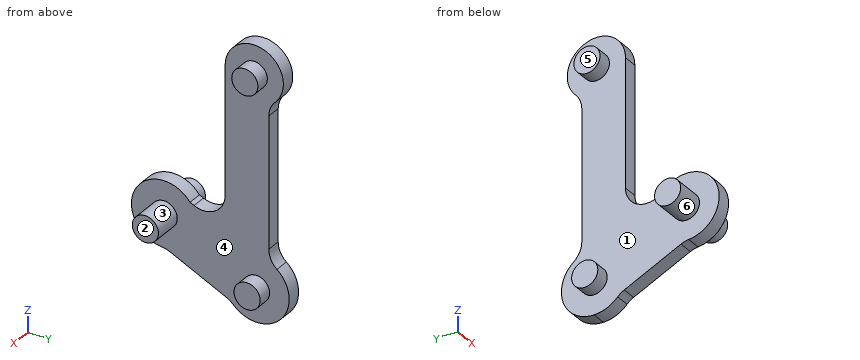
```python
from build123d import *

# Parameters (mm, degrees)
EXTRUDE_1_DEPTH     = 2
SKETCH_1_3_R        = 2
CUT_EXTRUDE_1_DEPTH = 35.66133887
FILLET_1_R          = 3
EXTRUDE_START       = -2
SKETCH_2_R          = 2
EXTRUDE_2_DEPTH     = 2
SKETCH_2_5_R        = 1.8
EXTRUDE_5_DEPTH     = 2
EXTRUDE_START_2     = -4
SKETCH_2_6_R        = 1.8
EXTRUDE_6_DEPTH     = 2
SKETCH_2_7_R        = 1.8
EXTRUDE_7_DEPTH     = 4
EXTRUDE_START_3     = -6
SKETCH_2_8_R        = 1.8
EXTRUDE_8_DEPTH     = 4


with BuildPart() as part:
    # 草图1 → 凸台-拉伸1 (new body)
    with BuildSketch(Plane(origin=(0, 0, 0), x_dir=(0, 0, -1), z_dir=(1, 0, 0))):
        with BuildLine():
            Line((-25, -6), (-25, 0))
            Line((-25, 0), (-21.535898385, 0))
            ThreePointArc((-21.535898385, 0), (-28.464101615, 0), (-25, -6))
        make_face()
        with BuildLine():
            Line((-21.535898385, 0), (-25, 0))
            Line((-25, 0), (-25, -6))
            ThreePointArc((-25, -6), (-22.171572875, -4.828427125), (-21, -2))
            ThreePointArc((-21, -2), (-21.136296695, -0.96472382), (-21.535898385, 0))
        make_face()
        with BuildLine():
            Line((-0.545176611, 0), (-21.535898385, 0))
            ThreePointArc((-21.535898385, 0), (-21.136296695, -0.96472382), (-21, -2))
            ThreePointArc((-21, -2), (-22.171572875, -4.828427125), (-25, -6))
            Line((-25, -6), (-2.797845949, -6))
            Line((-2.797845949, -6), (-0.871249866, -1.868401368))
            ThreePointArc((-0.871249866, -1.868401368), (-0.807766841, -0.916826597), (-0.545176611, 0))
        make_face()
        with BuildLine():
            ThreePointArc((8.125231148, -1.690473047), (4.486383017, 2.726360373), (-0.545176611, 0))
            Line((-0.545176611, 0), (0, 0))
            Line((0, 0), (7.250462296, -3.380946094))
            Line((7.250462296, -3.380946094), (6.37921243, -5.249347462))
            ThreePointArc((6.37921243, -5.249347462), (7.66521356, -3.67252807), (8.125231148, -1.690473047))
        make_face()
        with BuildLine():
            Line((0, 0), (-0.545176611, 0))
            ThreePointArc((-0.545176611, 0), (-0.807766841, -0.916826597), (-0.871249866, -1.868401368))
            Line((-0.871249866, -1.868401368), (0, 0))
        make_face()
        with BuildLine():
            Line((-0.871249866, -1.868401368), (-2.797845949, -6))
            Line((-2.797845949, -6), (0, -6))
            Line((0, -6), (0, -4.356499889))
            ThreePointArc((0, -4.356499889), (-0.621910323, -3.177681615), (-0.871249866, -1.868401368))
        make_face()
        with BuildLine():
            Line((0, -6), (-2.797845949, -6))
            Line((-2.797845949, -6), (-5.045405798, -10.819907651))
            ThreePointArc((-5.045405798, -10.819907651), (-0.389642338, -10.300397024), (2.205056498, -14.200853745))
            Line((2.205056498, -14.200853745), (6.37921243, -5.249347462))
            ThreePointArc((6.37921243, -5.249347462), (3.001481776, -6.147034134), (0, -4.356499889))
            Line((0, -4.356499889), (0, -6))
        make_face()
        with BuildLine():
            Line((7.250462296, -3.380946094), (0, 0))
            Line((0, 0), (0, -4.356499889))
            ThreePointArc((0, -4.356499889), (3.001481776, -6.147034134), (6.37921243, -5.249347462))
            Line((6.37921243, -5.249347462), (7.250462296, -3.380946094))
        make_face()
        with BuildLine():
            Line((0, -4.356499889), (0, 0))
            Line((0, 0), (-0.871249866, -1.868401368))
            ThreePointArc((-0.871249866, -1.868401368), (-0.621910323, -3.177681615), (0, -4.356499889))
        make_face()
        with BuildLine():
            ThreePointArc((2.205056498, -14.200853745), (-0.389642338, -10.300397024), (-5.045405798, -10.819907651))
            Line((-5.045405798, -10.819907651), (-5.916655664, -12.688309019))
            Line((-5.916655664, -12.688309019), (1.333806632, -16.069255112))
            Line((1.333806632, -16.069255112), (2.205056498, -14.200853745))
        make_face()
        with BuildLine():
            Line((-5.916655664, -12.688309019), (-5.045405798, -10.819907651))
            ThreePointArc((-5.045405798, -10.819907651), (-4.27347954, -18.418764477), (2.208575484, -14.378782065))
            ThreePointArc((2.208575484, -14.378782065), (2.207695651, -14.289800508), (2.205056498, -14.200853745))
            Line((2.205056498, -14.200853745), (1.333806632, -16.069255112))
            Line((1.333806632, -16.069255112), (-5.916655664, -12.688309019))
        make_face()
    extrude(amount=EXTRUDE_1_DEPTH)

    # 草图1<3> → 切除-拉伸1 (cut, through all)
    with BuildSketch(Plane(origin=(0, 0, 0), x_dir=(0, 0, -1), z_dir=(1, 0, 0))):
        with Locations((-25, -2)):
            Circle(SKETCH_1_3_R)
        with Locations((3.625231148, -1.690473047)):
            Circle(SKETCH_1_3_R)
        with Locations((-2.291424516, -14.378782065)):
            Circle(SKETCH_1_3_R)
    extrude(amount=CUT_EXTRUDE_1_DEPTH, mode=Mode.SUBTRACT)

    # 圆角1
    fillet_1_edges = [part.edges().sort_by_distance(p)[0] for p in [
        (1, -6, 2.797845949),
        (1, 0, 0.545176611),
        (1, -5.249347462, -6.37921243),
        (1, -14.200853745, -2.205056498),
        (1, 0, 21.535898385),
    ]]
    fillet(fillet_1_edges, radius=FILLET_1_R)

    # 草图2 → 凸台-拉伸2 (add)
    with BuildSketch(Plane(origin=(2, 0, 0), x_dir=(0, 0, -1), z_dir=(1, 0, 0)).offset(EXTRUDE_START)):
        with Locations((3.625231148, -1.690473047)):
            Circle(SKETCH_2_R)
        with Locations((-2.291424516, -14.378782065)):
            Circle(SKETCH_2_R)
        with Locations((-25, -2)):
            Circle(SKETCH_2_R)
    extrude(amount=EXTRUDE_2_DEPTH)

    # 草图2<5> → 凸台-拉伸5 (add)
    with BuildSketch(Plane(origin=(2, 0, 0), x_dir=(0, 0, -1), z_dir=(1, 0, 0))):
        with Locations((-25, -2)):
            Circle(SKETCH_2_5_R)
        with Locations((3.625231148, -1.690473047)):
            Circle(SKETCH_2_5_R)
    extrude(amount=EXTRUDE_5_DEPTH)

    # 草图2<6> → 凸台-拉伸6 (add)
    with BuildSketch(Plane(origin=(2, 0, 0), x_dir=(0, 0, -1), z_dir=(1, 0, 0)).offset(EXTRUDE_START_2)):
        with Locations((-25, -2)):
            Circle(SKETCH_2_6_R)
        with Locations((3.625231148, -1.690473047)):
            Circle(SKETCH_2_6_R)
    extrude(amount=EXTRUDE_6_DEPTH)

    # 草图2<7> → 凸台-拉伸7 (add)
    with BuildSketch(Plane(origin=(2, 0, 0), x_dir=(0, 0, -1), z_dir=(1, 0, 0))):
        with Locations((-2.291424516, -14.378782065)):
            Circle(SKETCH_2_7_R)
    extrude(amount=EXTRUDE_7_DEPTH)

    # 草图2<8> → 凸台-拉伸8 (add)
    with BuildSketch(Plane(origin=(2, 0, 0), x_dir=(0, 0, -1), z_dir=(1, 0, 0)).offset(EXTRUDE_START_3)):
        with Locations((-2.291424516, -14.378782065)):
            Circle(SKETCH_2_8_R)
    extrude(amount=EXTRUDE_8_DEPTH)


solid = part.part
```
Geometry check sheet. Reference: the model listing, model coordinates, mm. Face numbers are marked on the shaded views. A direction names the side the tool comes from. Give positions to 0.01 mm unless a question says otherwise; leave off trailing zeros. Order: outer loops, then holes, each group sorted by start corner. A loop starts at its lowest first (then second) coordinate and runs counter-clockwise, first axis right, second up.
1. Access from +Z, -Z, +X, -X, +Y, -Y to the whole of each face (thin tool, end or side, straight path). Record for the marked faces 5 and 6.
2. Thickness scan on L1, parallel to Y at x = 1.75, z = 20; L2, parallel to X at y = -5.25, z = 5; L3, parallel to X at y = -2, z = 24. Record the ranges inside material, lowest first.
3. Release check for a two-part mould opening along Z. For the marked faces 1, 2, 3 and 4 record: pulls with the +Z half, pulls with the -Z half, needs draft (parallel to the pull), parting line crosses it, or undercut.
4. Section check D-D, the plane z = 15.5. Enter the section's corners in (x, y), and give its area (3 significant figures).
5. Gauge pin test, flat ends, axial feed: pin 1 Ø2 at (x, z) = (4.5, 3.5) entering from -Y; pin 2 Ø1 at (y, z) = (-3.5, -4.5) entering from -X; pin 3 Ø4 at (x, z) = (1, -3.5) entering from -Y; pin 4 Ø1.5 at (x, y) = (-2.5, -5.5) entering from -Z. Record the tip position at first contact, or that the pin passes through.
6. Section check A-A, the plane z = 24. Enter the section's corners in (x, y), and give its area (3 significant figures).
7. Section check C-C, the plane x = -2.5. Enter the section's corners in (y, z).
8. Section check B-B, the plane x = 3.25. Enter the section's corners in (y, z).
Values follow:
1. face 5: +Z, -Z, -X, +Y, -Y
1. face 6: -X
2. L1: y = -6 to 0
2. L2: x = 0 to 2
2. L3: x = -2 to 4
3. face 1: undercut
3. face 2: needs draft
3. face 3: parting line crosses it
3. face 4: undercut
4. outline: (0, -6) - (2, -6) - (2, 0) - (0, 0) - close
4. area: 12.0 mm2
5. pin 1: stops at y = -16.17
5. pin 2: stops at x = -2
5. pin 3: stops at y = -16.8
5. pin 4: passes through
6. outline: (-2, -3.5) - (0, -3.5) - (0, -6) - (2, -6) - (2, -3.5) - (4, -3.5) - (4, -0.5) - (2, -0.5) - (2, 1.87) - (0, 1.87) - (0, -0.5) - (-2, -0.5) - close
6. area: 27.7 mm2
7. outline: circle Ø3.6 at (-14.38, 2.29)
8. outline: circle Ø3.6 at (-14.38, 2.29); circle Ø3.6 at (-2, 25); circle Ø3.6 at (-1.69, -3.63)
